For this review, use the dimensioned drawing (mm, ordinates from the lowest corner) and the shaded views. A direction names the side the tool comes from. Give positions to 0.01 mm unless a question says otherwise; leave off trailing zeros. Write each loop counter-clockwise with the first axis right and the second up, starting at its lowest first coordinate (ties: lowest second). Pieces come first, ordered by that corner, then holes. Notation, with made-up numbers: M 35,61 L 79,61 A10 ccw 79,74 Z; hole C -28.75,-8.5 d1. An arc over 180 degrees is marked long. Answer in a Markdown table with one row per item.
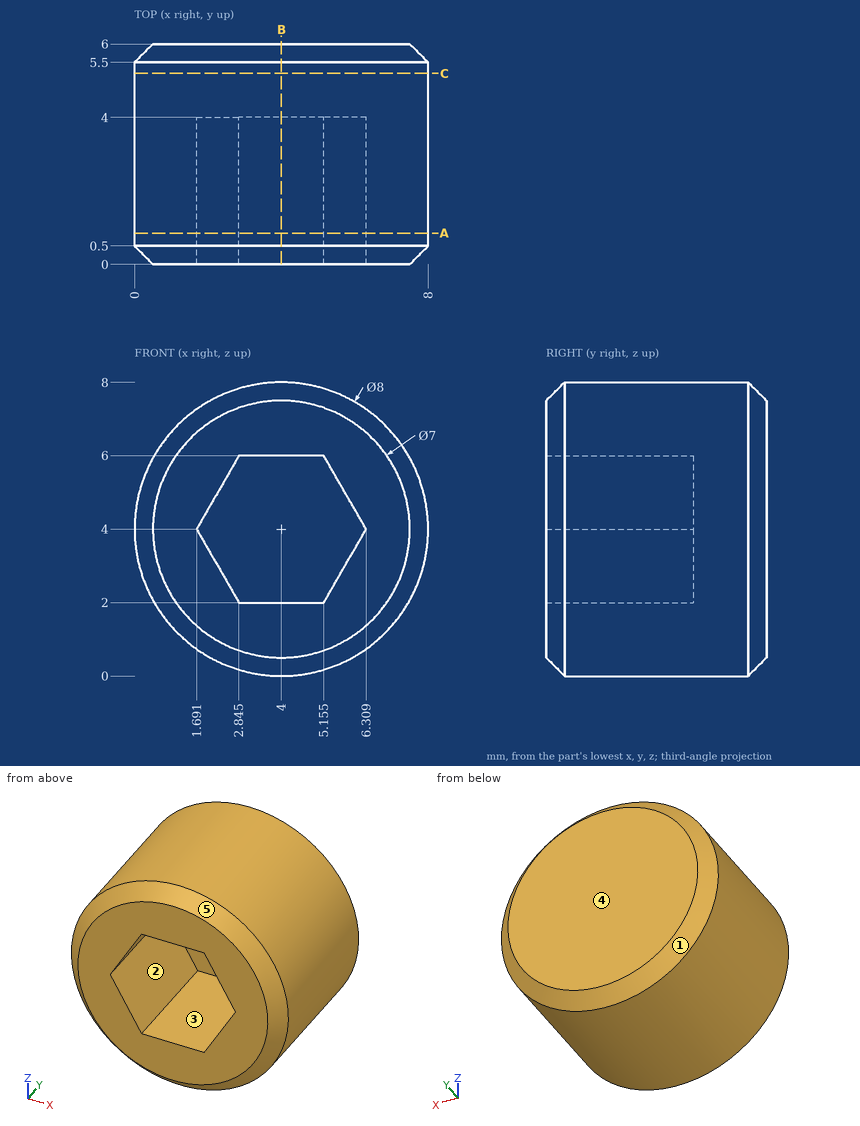
1) Add section B-B (x = 4). Write out the cut boundary in (y, z), and give its area (3 significant figures).
Geometry says:
| item | result |
|---|---|
| outline | M 0,0.5 L 0.5,0 L 5.5,0 L 6,0.5 L 6,7.5 L 5.5,8 L 0.5,8 L 0,7.5 L 0,6 L 4,6 L 4,2 L 0,2 Z |
| area | 31.5 mm^2 |
2) Add section A-A (y = 0.85). Write out the cut boundary in (x, z) (1 decimal), and give its area (3 significant figures).
Geometry says:
| item | result |
|---|---|
| outline | C 4,4 d8; hole M 1.7,4 L 2.8,2 L 5.2,2 L 6.3,4 L 5.2,6 L 2.8,6 Z |
| area | 36.4 mm^2 |
3) The part is to be moulded in two halves that separate along X. For the marked faces 3, 4 and 5, say which applies: released by +X, released by -X, zero draft, split by the parting line, or undercut.
Geometry says:
| item | result |
|---|---|
| face 3 | undercut |
| face 4 | zero draft |
| face 5 | split by the parting line |
4) For the marked faces 1 and 2, list the 3-axis set-ups (+Z, -Z, +X, -X, +Y, -Y) from which the entire face can be reached by the end or side of a thin tool; tool diameter is ignored.
Geometry says:
| item | result |
|---|---|
| face 1 | +Y |
| face 2 | -Y |
5) To check wall thickness, follow probe 1 along Y at (x, z) = (6, 4); probe 2 along Z at (x, y) = (4.5, 0.8); probe 3 along X at (y, z) = (0.55, 4.5). State the ranges of each line that lie inside material, in increasing order. Write a range as [from, to].
Geometry says:
| item | result |
|---|---|
| probe 1 | [4, 6] |
| probe 2 | [0.03, 2], [6, 7.97] |
| probe 3 | [0.03, 1.98], [6.02, 7.97] |
6) Add section C-C (y = 5.2). Write out the cut boundary in (x, z).
Geometry says:
| item | result |
|---|---|
| outline | C 4,4 d8 |
7) Insertion check: P1, Ø4, axis at x = 2.5, z = 6.5, coming from the -Y side; P2, Ø1, axis at x = 3, y = 4, coming from the +Z side; P3, Ø2, axis at x = 4, z = 4.5, coming from the -Y side. Each pin has a flat end and moves straight along its axis. Give the tip position at first contact, or say it passes through.
Geometry says:
| item | result |
|---|---|
| P1 | y = 0 |
| P2 | z = 7.97 |
| P3 | y = 4 |
